Geometry: see drawing. Coordinates: mm, zero at the bounding-box minimum. A direction names the side the tool comes from. Round coordinates to 2 decimals unless told otherwise and drop trailing zeros. Order: outer loops, then holes, each group sorted by start corner. A loop starts at its lowest first (then second) coordinate and runs counter-clockwise, first axis right, second up.
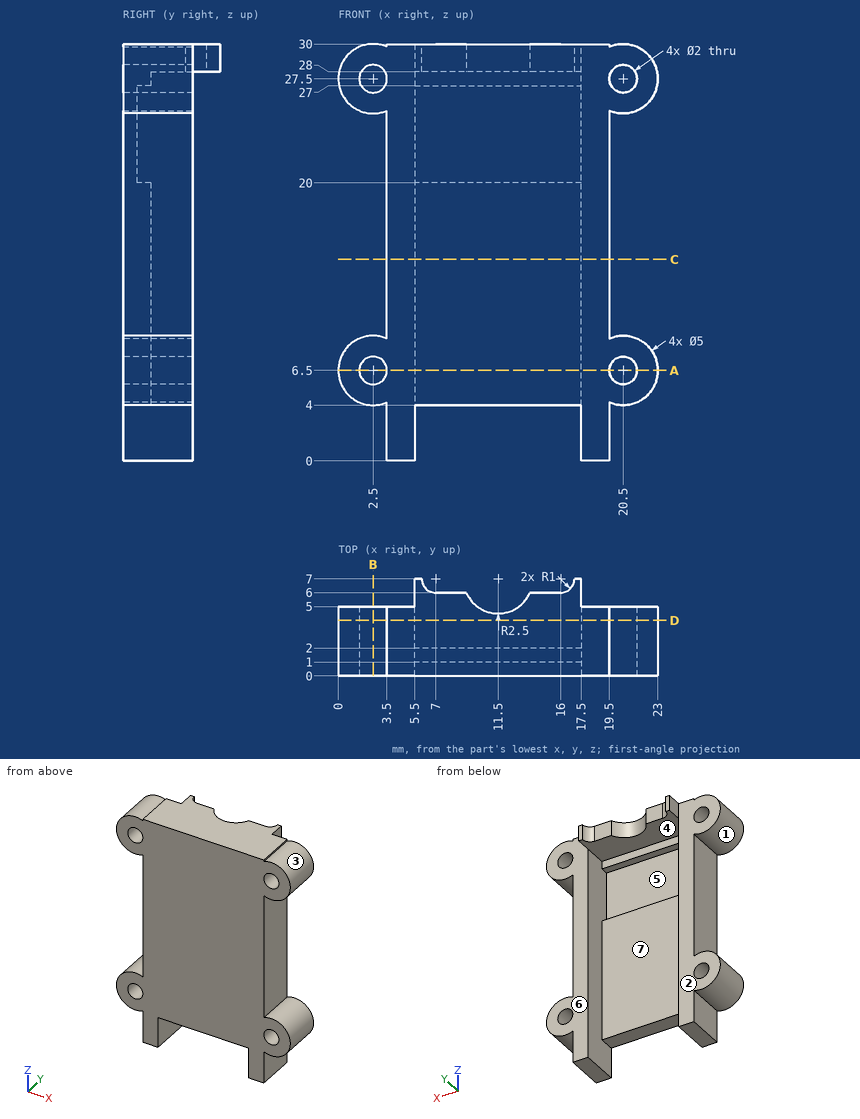
1. First-contact query: pin 1 (1 mm diameter, centred on x = 7.5, z = 29, fed in from +Y); pin 2 (1.5 mm diameter, centred on x = 15.5, y = 4.5, fed in from -Z); pin 3 (2 mm diameter, centred on y = 3.5, z = 15, fed in from -X); pin 4 (1 mm diameter, centred on x = 18, y = 1.5, fed in from -Z). Flat tips, straight axial feed; report the tip coordinate or a pass-through.
2. Section B-B on x = 2.5. Return loops of the section in (y, z).
3. Pull-direction query (Z, two-part tool) for the marked faces 1, 2, 3 and 4; classes: released by +Z, released by -Z, zero draft, split by the parting line, or undercut.
4. Access query for the marked faces 5, 6 and 7. Directions: +Z, -Z, +X, -X, +Y, -Y. A direction counts if a zero-diameter tool reaches every point of the face in a straight line with its end or side. Return the directions, or none.
5. Section C-C on z = 14.5. Return loops of the section in (x, y).
6. Section D-D on y = 4. Return loops of the section in (x, z), plus the area to 3 significant figures.
7. Line query: line 1 along Z through (x, y) = (20.5, 2.1); line 2 along X through (y, z) = (3.5, 14); line 3 along Z through (x, y) = (21.25, 2.25). Output: solid intervals per line, ascending.
8. Section A-A on z = 6.5. Return loops of the section in (x, y).
Result:
1. pin 1: stops at y = 6
1. pin 2: stops at z = 28
1. pin 3: stops at x = 3.5
1. pin 4: stops at z = 0
2. outline: (0, 4) - (5, 4) - (5, 5.5) - (0, 5.5) - close; (0, 7.5) - (5, 7.5) - (5, 9) - (0, 9) - close; (0, 25) - (5, 25) - (5, 26.5) - (0, 26.5) - close; (0, 28.5) - (5, 28.5) - (5, 30) - (0, 30) - close
3. face 1: undercut
3. face 2: zero draft
3. face 3: undercut
3. face 4: released by -Z
4. face 5: +Y
4. face 6: +Z, -Z, +X, +Y
4. face 7: -Z, +Y
5. outline: (3.5, 0) - (19.5, 0) - (19.5, 5) - (17.5, 5) - (17.5, 2) - (5.5, 2) - (5.5, 5) - (3.5, 5) - close
6. outline: (3.5, 0) - (5.5, 0) - (5.5, 28) - (17.5, 28) - (17.5, 0) - (19.5, 0) - (19.5, 4.21) arc R2.5 ccw (long way) to (19.5, 8.79) - (19.5, 25.21) arc R2.5 ccw (long way) to (19.5, 29.79) - (19.5, 30) - (3.5, 30) - (3.5, 29.79) arc R2.5 ccw (long way) to (3.5, 25.21) - (3.5, 8.79) arc R2.5 ccw (long way) to (3.5, 4.21) - close; hole circle Ø2 at (2.5, 6.5); hole circle Ø2 at (2.5, 27.5); hole circle Ø2 at (20.5, 6.5); hole circle Ø2 at (20.5, 27.5)
6. area: 190 mm2
7. line 1: z = 4 to 5.5, 7.5 to 9, 25 to 26.5, 28.5 to 30
7. line 2: x = 3.5 to 5.5, 17.5 to 19.5
7. line 3: z = 4.12 to 5.84, 7.16 to 8.88, 25.12 to 26.84, 28.16 to 29.88
8. outline: (0, 0) - (1.5, 0) - (1.5, 5) - (0, 5) - close; (3.5, 0) - (19.5, 0) - (19.5, 5) - (17.5, 5) - (17.5, 2) - (5.5, 2) - (5.5, 5) - (3.5, 5) - close; (21.5, 0) - (23, 0) - (23, 5) - (21.5, 5) - close
